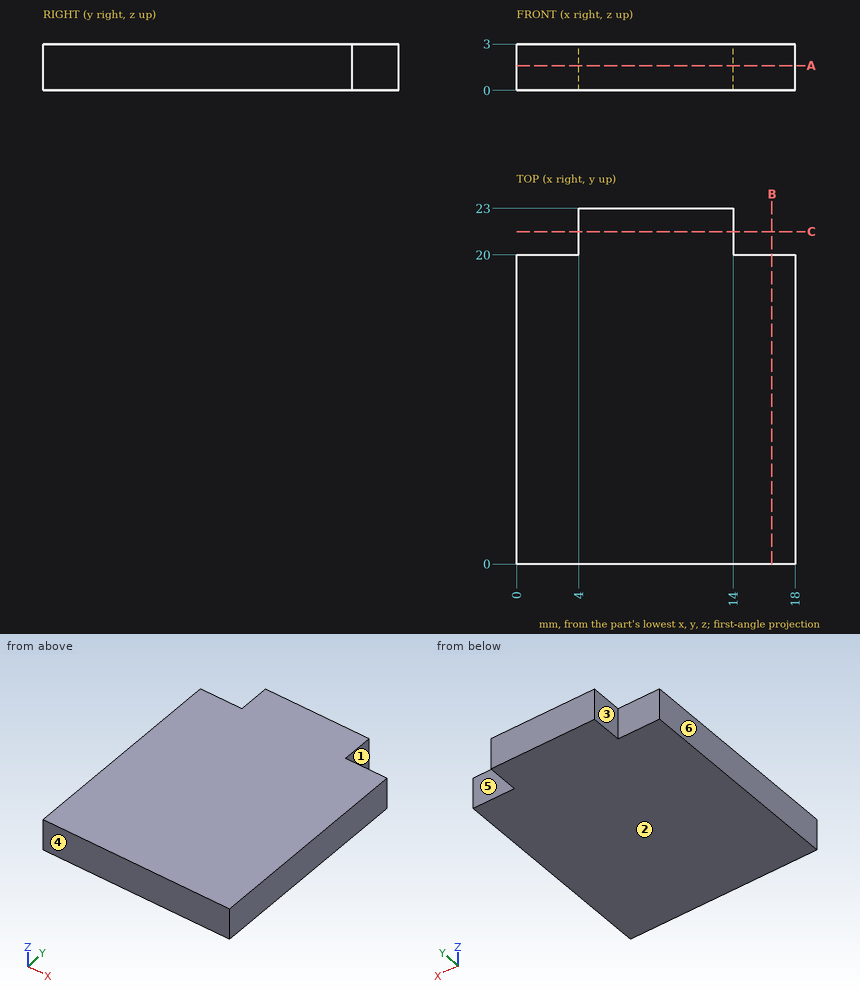
Input: dimensioned drawing with shaded views. Units: mm. Origin: part minimum x, y, z. A direction names the side the tool comes from. Coordinates: 2 decimals unless noted, no trailing zeros. Loops run counter-clockwise (first coordinate to the right, second up) from the corner with the lowest first, then second, coordinate; pieces in that order, holes last.
Q1. Set-up query: the marked faces 1, 2 and 3. Return all of +Z, -Z, +X, -X, +Y, -Y with unobstructed straight access to the full face (end or side cutting, diameter ignored); none if empty.
Results are:
face 1: +Z, -Z, +X, +Y
face 2: -Z, +X, -X, +Y, -Y
face 3: +Z, -Z, -X, +Y
Q2. Mould query, pull axis Y, two halves, no side actions, for the marked faces 4, 5 and 6. Classes: +Y half, -Y half, draft (parallel to the pull), parting line (faces both ways), or undercut.
Results are:
face 4: -Y half
face 5: +Y half
face 6: draft
Q3. Section A-A, the plane z = 1.6. Return the cut outline in (x, y).
Results are:
outline: (0, 0) - (18, 0) - (18, 20) - (14, 20) - (14, 23) - (4, 23) - (4, 20) - (0, 20) - close
Q4. Section C-C, the plane y = 21.5. Return the cut outline in (x, z).
Results are:
outline: (4, 0) - (14, 0) - (14, 3) - (4, 3) - close
Q5. Section B-B, the plane x = 16.5. Return the cut outline in (y, z), and give its area (3 significant figures).
Results are:
outline: (0, 0) - (20, 0) - (20, 3) - (0, 3) - close
area: 60.0 mm2
Q6. Line query: line 1 along Y through (x, z) = (16.25, 2.95). Output: solid intervals per line, ascending.
Results are:
line 1: y = 0 to 20
